CAD build for the part. Positions are in the model's coordinates, mm. Round coordinates to 2 decimals unless told otherwise and drop trailing zeros. Order: outer loops, then holes, each group sorted by start corner. A loop starts at its lowest first (then second) coordinate and runs counter-clockwise, first axis right, second up. Notation, with made-up numbers: M -34.75,-18.5 L -5.75,-18.5 A28 cw -5.75,1.5 Z; hole C -34,45 d4. An arc over 180 degrees is marked long. Put each result on its own line as item: value.
```python
from build123d import *

# Parameters (mm, degrees)
BOSS_EXTRUDE1_DEPTH      = 37
BOSS_EXTRUDE1_DEPTH_BACK = 37
FILLET1_R                = 0.1
M2X0_4_TAPPED_HOLE1_D    = 1.6


with BuildPart() as part:
    # Sketch1 → Boss-Extrude1 (new, two sides: drawn at the far end of the back side and taken through both)
    with BuildSketch(Plane(origin=(0, 0, 0), x_dir=(0, 0, -1), z_dir=(1, 0, 0)).offset(-BOSS_EXTRUDE1_DEPTH_BACK)):
        Polygon((0, -3.2), (-2, -1.2), (-2, 3.2), (0, 3.2), align=None)
    extrude(amount=BOSS_EXTRUDE1_DEPTH + BOSS_EXTRUDE1_DEPTH_BACK)

    # Fillet1
    fillet1_edges = [part.edges().sort_by_distance(p)[0] for p in [
        (-37, -2.2, 1),
        (-37, 0, 0),
        (0, 3.2, 2),
        (0, -1.2, 2),
        (37, -2.2, 1),
        (37, 0, 0),
        (37, 3.2, 1),
        (37, 1, 2),
        (0, -3.2, 0),
        (0, 3.2, 0),
        (-37, 3.2, 1),
        (-37, 1, 2),
    ]]
    fillet(fillet1_edges, radius=FILLET1_R)

    # M2x0.4 Tapped Hole1 (through all)
    with Locations(Plane.XY.offset(2)):
        with Locations((22, 0), (0, 0), (-22, 0)):
            Hole(M2X0_4_TAPPED_HOLE1_D / 2)


solid = part.part
```
Item 1: Band-saw the part on A-A on x = -22. Give the cut face in (y, z).
Answers below:
outline: M -3.03,0.17 A0.1 ccw -2.96,0 L -0.8,0 L -0.8,2 L -1.16,2 A0.1 ccw -1.23,1.97 Z; M 0.8,0 L 3.1,0 A0.1 ccw 3.2,0.1 L 3.2,1.9 A0.1 ccw 3.1,2 L 0.8,2 Z
Item 2: Mould opens along Y. For faces 1 (the flat face through (37, 1, 1)), 2 (the cylindrical face through (-21.41, 0.54, 0.99)), 3 (the flat face through (-0.5, -2.1, 1.1)), 4 (the cylindrical face through (22.59, 0.54, 0.99)) say: pulls with the +Y half, pulls with the -Y half, needs draft (parallel to the pull), parting line crosses it, or undercut.
Answers below:
face 1: needs draft
face 2: undercut
face 3: pulls with the -Y half
face 4: undercut
Item 3: Probe line 1 along X through (y, z) = (-0.5, 1.35); line 2 along X through (y, z) = (0.25, 1.7); line 3 along Y through (x, z) = (22, 0.7). List the from-to ranges inside material, lowest first. Write a range as [from, to].
Answers below:
line 1: [-37, -22.62], [-21.38, -0.62], [0.62, 21.38], [22.62, 37]
line 2: [-37, -22.76], [-21.24, -0.76], [0.76, 21.24], [22.76, 37]
line 3: [-2.5, -0.8], [0.8, 3.2]
Item 4: Band-saw the part on B-B on y = 0. Give the cut face in (x, z), and give its area (3 significant figures).
Answers below:
outline: M -37,0.1 A0.1 ccw -36.9,0 L -22.8,0 L -22.8,2 L -36.9,2 A0.1 ccw -37,1.9 Z; M -21.2,0 L -0.8,0 L -0.8,2 L -21.2,2 Z; M 0.8,0 L 21.2,0 L 21.2,2 L 0.8,2 Z; M 22.8,0 L 36.9,0 A0.1 ccw 37,0.1 L 37,1.9 A0.1 ccw 36.9,2 L 22.8,2 Z
area: 138 mm²
Item 5: Band-saw the part on C-C on x = -4. Give the cut face in (y, z).
Answers below:
outline: M -3.03,0.17 A0.1 ccw -2.96,0 L 3.1,0 A0.1 ccw 3.2,0.1 L 3.2,1.9 A0.1 ccw 3.1,2 L -1.16,2 A0.1 ccw -1.23,1.97 Z
Item 6: Pin check, flat tip, straight feed: P1, Ø1.4, axis at x = 0, y = 0, coming from the -Z side. Stop position of the tip, or through.
Answers below:
P1: through
Item 7: Band-saw the part on D-D on z = 0.55. State how many separate pieces and enclosed holes the cut face has, and give its area (3 significant figures).
Answers below:
separate pieces: 1
enclosed holes: 3
area: 427 mm²
